Geometry check sheet. Reference: the model listing, model coordinates, mm. A direction names the side the tool comes from. Round coordinates to 2 decimals unless told otherwise and drop trailing zeros. Order: outer loops, then holes, each group sorted by start corner. A loop starts at its lowest first (then second) coordinate and runs counter-clockwise, first axis right, second up. Notation, with made-up numbers: (71, 21) - (86, 21) arc R31 ccw to (86, 45) - close; hole circle Ø6 at (76, 10.5). An arc over 180 degrees is marked (long way). Use a Markdown table: item, result. Add a question column.
(1) Gauge pin test, flat ends, axial feed: P1, Ø8, axis at x = -16, y = -1, coming from the +Z side; P2, Ø12, axis at x = 9.5, z = -24, coming from the -Y side; P3, Ø1.5, axis at x = -20.5, z = -28, coming from the +Y side; P4, Ø1.5, axis at y = 5.5, z = -14.5, coming from the -X side. Record the tip position at first contact, or that the pin passes through.
(2) Section check C-C on y = 5. Record the boundary of the cut face in (x, z), then the cut area to 3 significant figures.
(3) Section check A-A on z = -27. Record the boundary of the cut face in (x, y), then the cut area to 4 significant figures.
(4) Section check B-B on x = -45.5. Record the boundary of the cut face in (y, z).
(5) Access from +Z, -Z, +X, -X, +Y, -Y to the whole of each face (thin tool, end or side, straight path). Record for faces 1 (the face through (0, -4, -17)), 2 (the face through (-65, 1, -21)), 3 (the face through (-58, 4, -7)).
(6) Section check D-D on z = -12. Record the boundary of the cut face in (x, y), then the cut area to 4 significant figures.
(7) Thickness scan on line 1 along X through (y, z) = (-3.5, -18); line 2 along Y through (x, z) = (-10.5, -32.5); line 3 along Y through (x, z) = (-19.5, -11). Record the ranges inside material, lowest first. Write a range as [from, to].
```python
from build123d import *

# Parameters (mm, degrees)
BOSS_EXTRUDE1_DEPTH = 35
CUT_EXTRUDE1_DEPTH  = 20


with BuildPart() as part:
    # Sketch1 → Boss-Extrude1 (new body)
    with BuildSketch(Plane.XY):
        Polygon((0, 0), (0, -8), (-65, -8), (-65, 4), (-65, 24), (-40, 24), (-23, 24), (15, 9), (15, 0), align=None)
    extrude(amount=-BOSS_EXTRUDE1_DEPTH)

    # Sketch2 → Cut-Extrude1 (cut)
    with BuildSketch(Plane(origin=(0, 24, 0), x_dir=(1, 0, 0), z_dir=(0, 1, 0))):
        Polygon((-40, 0), (-65, 25), (-65, 0), align=None)
    extrude(amount=-CUT_EXTRUDE1_DEPTH, mode=Mode.SUBTRACT)


solid = part.part
```
Check sheet entries:
| question | item | result |
|---|---|---|
| 1 | P1 | stops at z = 0 |
| 1 | P2 | stops at y = 0 |
| 1 | P3 | stops at y = 23.31 |
| 1 | P4 | stops at x = -55.25 |
| 2 | outline | (-65, -35) - (15, -35) - (15, 0) - (-40, 0) - (-65, -25) - close |
| 2 | area | 2,490 mm2 |
| 3 | outline | (-65, -8) - (0, -8) - (0, 0) - (15, 0) - (15, 9) - (-23, 24) - (-65, 24) - close |
| 3 | area | 2,155 mm2 |
| 4 | outline | (-8, -35) - (24, -35) - (24, -5.5) - (4, -5.5) - (4, 0) - (-8, 0) - close |
| 5 | face 1 | +Z, -Z, +X, -Y |
| 5 | face 2 | +Z, -Z, -X, +Y, -Y |
| 5 | face 3 | +Z, -X, +Y |
| 6 | outline | (-65, -8) - (0, -8) - (0, 0) - (15, 0) - (15, 9) - (-23, 24) - (-52, 24) - (-52, 4) - (-65, 4) - close |
| 6 | area | 1,895 mm2 |
| 7 | line 1 | x = [-65, 0] |
| 7 | line 2 | y = [-8, 19.07] |
| 7 | line 3 | y = [-8, 22.62] |
